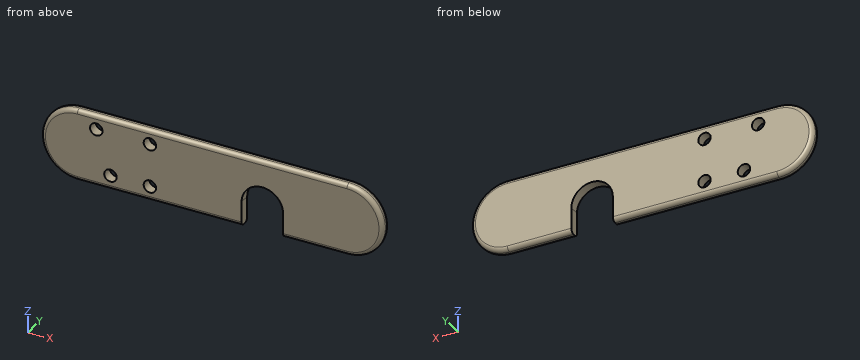
from build123d import *

# Parameters (mm, degrees)
BOSS_EXTRUDE1_DEPTH = 2.5
CUT_EXTRUDE1_REACH  = 86.406
SKETCH2_R           = 3
FILLET1_R           = 2
CUT_EXTRUDE2_DEPTH  = 10


with BuildPart() as part:
    # Sketch1 → Boss-Extrude1 (new, symmetric)
    with BuildSketch(Plane(origin=(0, 0, 0), x_dir=(1, 0, 0), z_dir=(0, 1, 0))):
        with BuildLine():
            Line((-65.005, 17.43), (65.005, 17.43))
            ThreePointArc((65.005, 17.43), (82.435, 0), (65.005, -17.43))
            Line((65.005, -17.43), (-65.005, -17.43))
            ThreePointArc((-65.005, -17.43), (-82.435, 0), (-65.005, 17.43))
        make_face()
    extrude(amount=BOSS_EXTRUDE1_DEPTH, both=True)

    # Sketch2 → Cut-Extrude1 (cut, up to next)
    with BuildSketch(Plane(origin=(0, 2.5, 0), x_dir=(1, 0, 0), z_dir=(0, 1, 0)), mode=Mode.PRIVATE) as cut_extrude1_sk1:
        with Locations(Location((-49.065, 10.43, 0), (0, 0, 270))):
            Circle(SKETCH2_R)
    cut_extrude1_tool1 = extrude(cut_extrude1_sk1.sketch, amount=-CUT_EXTRUDE1_REACH, mode=Mode.PRIVATE) & part.part
    # Sketch2 → Cut-Extrude1 (cut, up to next)
    with BuildSketch(Plane(origin=(0, 2.5, 0), x_dir=(1, 0, 0), z_dir=(0, 1, 0)), mode=Mode.PRIVATE) as cut_extrude1_sk2:
        with Locations(Location((-30.035, 10.43, 0), (0, 0, 270))):
            Circle(SKETCH2_R)
    cut_extrude1_tool2 = extrude(cut_extrude1_sk2.sketch, amount=-CUT_EXTRUDE1_REACH, mode=Mode.PRIVATE) & part.part
    # Sketch2 → Cut-Extrude1 (cut, up to next)
    with BuildSketch(Plane(origin=(0, 2.5, 0), x_dir=(1, 0, 0), z_dir=(0, 1, 0)), mode=Mode.PRIVATE) as cut_extrude1_sk3:
        with Locations(Location((-55.895, -10.43, 0), (0, 0, 270))):
            Circle(SKETCH2_R)
    cut_extrude1_tool3 = extrude(cut_extrude1_sk3.sketch, amount=-CUT_EXTRUDE1_REACH, mode=Mode.PRIVATE) & part.part
    # Sketch2 → Cut-Extrude1 (cut, up to next)
    with BuildSketch(Plane(origin=(0, 2.5, 0), x_dir=(1, 0, 0), z_dir=(0, 1, 0)), mode=Mode.PRIVATE) as cut_extrude1_sk4:
        with Locations(Location((-30.035, -10.43, 0), (0, 0, 270))):
            Circle(SKETCH2_R)
    cut_extrude1_tool4 = extrude(cut_extrude1_sk4.sketch, amount=-CUT_EXTRUDE1_REACH, mode=Mode.PRIVATE) & part.part
    add(cut_extrude1_tool1.solids().sort_by_distance((-49.065, 2.5, -10.43))[0], mode=Mode.SUBTRACT)
    add(cut_extrude1_tool2.solids().sort_by_distance((-30.035, 2.5, -10.43))[0], mode=Mode.SUBTRACT)
    add(cut_extrude1_tool3.solids().sort_by_distance((-55.895, 2.5, 10.43))[0], mode=Mode.SUBTRACT)
    add(cut_extrude1_tool4.solids().sort_by_distance((-30.035, 2.5, 10.43))[0], mode=Mode.SUBTRACT)

    # Fillet1
    fillet1_edges = [part.edges().sort_by_distance(p)[0] for p in [
        (82.435, 2.5, 0),
        (0, 2.5, -17.43),
        (-82.435, 2.5, 0),
        (0, -2.5, -17.43),
        (82.435, -2.5, 0),
        (0, -2.5, 17.43),
        (-82.435, -2.5, 0),
        (0, 2.5, 17.43),
    ]]
    fillet(fillet1_edges, radius=FILLET1_R)

    # Sketch3 → Cut-Extrude2 (cut)
    with BuildSketch(Plane(origin=(0, 2.5, 0), x_dir=(1, 0, 0), z_dir=(0, 1, 0))):
        with BuildLine():
            Line((34.165, 17.43), (34.165, 5.43))
            ThreePointArc((34.165, 5.43), (24.165, -4.57), (14.165, 5.43))
            Line((14.165, 5.43), (14.165, 17.43))
            Line((14.165, 17.43), (34.165, 17.43))
        make_face()
    extrude(amount=-CUT_EXTRUDE2_DEPTH, mode=Mode.SUBTRACT)


solid = part.part
For this review, take the finished solid that the model builds, in its own axes (mm). Give positions to 0.01 mm unless a question says otherwise; leave off trailing zeros. Loops run counter-clockwise (first coordinate to the right, second up) from the corner with the lowest first, then second, coordinate; pieces in that order, holes last.
Item 1: For line 1 along Z through (x, y) = (-30, 0.8); line 2 along X through (y, z) = (-0.5, 10.43) (3 decimals); line 3 along Z through (x, y) = (-32.5, -1.75), list the stretches that pass through material, from the lowest coordinate up.
Item 2: Take a section at C-C, the plane y = 1.45. State the section outline as (x, z) points (3 decimals), and give its area (3 significant figures).
Item 3: Take a section at A-A, the plane z = 0. State the section outline as (x, y) points (3 decimals), and give its area (3 significant figures).
Item 4: Take a section at B-B, the plane x = -2. State the section outline as (y, z) points.
Item 5: Take a section at D-D, the plane z = 10.5. Give the number of separate pieces and of enclosed holes in the cut face, and give its area (3 significant figures).
Item 6: Insertion check: pin 1 (3 mm diameter, centred on y = -0.5, z = 11.5, fed in from -X); pin 2 (2.5 mm diameter, centred on y = -0.5, z = -11.5, fed in from +X); pin 3 (2 mm diameter, centred on y = 0.5, z = 5, fed in from +X). Each pin has a flat end and moves straight along its axis. Give the tip position at first contact, or say it passes through.
Calculated:
1. line 1: z = -17.41 to -13.43, -7.43 to 7.43, 13.43 to 17.41
1. line 2: x = -78.97 to -58.895, -52.895 to -33.035, -27.035 to 78.97
1. line 3: z = -16.99 to -12.14, -8.72 to 8.72, 12.14 to 16.99
2. outline: (-65.005, -17.19) - (14.165, -17.19) - (14.165, -5.43) arc R10 cw to (34.165, -5.43) - (34.165, -17.19) - (65.005, -17.19) arc R17.19 ccw to (65.005, 17.19) - (-65.005, 17.19) arc R17.19 ccw to start; hole circle Ø6 at (-55.895, 10.43); hole circle Ø6 at (-49.065, -10.43); hole circle Ø6 at (-30.035, -10.43); hole circle Ø6 at (-30.035, 10.43)
2. area: 4,890 mm2
3. outline: (-82.435, -0.5) arc R2 ccw to (-80.435, -2.5) - (15.768, -2.5) - (15.768, 2.5) - (-80.435, 2.5) arc R2 ccw to (-82.435, 0.5) - close; (32.562, -2.5) - (80.435, -2.5) arc R2 ccw to (82.435, -0.5) - (82.435, 0.5) arc R2 ccw to (80.435, 2.5) - (32.562, 2.5) - close
3. area: 737 mm2
4. outline: (-2.5, -15.43) arc R2 ccw to (-0.5, -17.43) - (0.5, -17.43) arc R2 ccw to (2.5, -15.43) - (2.5, 15.43) arc R2 ccw to (0.5, 17.43) - (-0.5, 17.43) arc R2 ccw to (-2.5, 15.43) - close
5. separate pieces: 3
5. enclosed holes: 0
5. area: 725 mm2
6. pin 1: stops at x = -79.28
6. pin 2: stops at x = 79.1
6. pin 3: stops at x = 81.97
